```python
from build123d import *

# Parameters (mm, degrees)
STEEL_TUBE_STOCK_SKETCH_W        = 20
STEEL_TUBE_STOCK_SKETCH_H        = 55
STEEL_TUBE_STOCK_DEPTH           = 40
TUBE_INTERIOR_SKETCH_W           = 16
TUBE_INTERIOR_SKETCH_H           = 55.2
TUBE_INTERIOR_DEPTH              = 36
GUIDE_BUSH_CLEARANCE_1_SKETCH_R  = 6.2
GUIDE_BUSH_CLEARANCE_1_DEPTH     = 20.3
GUIDE_BUSH_CLEARANCE_2_SKETCH_R  = 6.2
GUIDE_BUSH_CLEARANCE_2_DEPTH     = 20.3
SCREW_THROUGH_CLEARANCE_SKETCH_R = 3.3
SCREW_THROUGH_CLEARANCE_DEPTH    = 20.3
SPRING_PIN_CLEARANCE_1_SKETCH_R  = 1.7
SPRING_PIN_CLEARANCE_1_DEPTH     = 2.2
SPRING_PIN_CLEARANCE_2_SKETCH_R  = 1.7
SPRING_PIN_CLEARANCE_2_DEPTH     = 2.2
SPRING_PIN_CLEARANCE_3_SKETCH_R  = 1.7
SPRING_PIN_CLEARANCE_3_DEPTH     = 2.2
CLAMP_BOLT_CLEARANCE_1_SKETCH_R  = 1.7
CLAMP_BOLT_CLEARANCE_1_DEPTH     = 2.3
CLAMP_BOLT_CLEARANCE_2_SKETCH_R  = 1.7
CLAMP_BOLT_CLEARANCE_2_DEPTH     = 2.3


with BuildPart() as part:
    # Steel tube stock sketch → Steel tube stock (new body)
    with BuildSketch(Plane.XY.offset(-29)):
        with Locations((39.708348754, -28.5)):
            Rectangle(STEEL_TUBE_STOCK_SKETCH_W, STEEL_TUBE_STOCK_SKETCH_H)
    extrude(amount=STEEL_TUBE_STOCK_DEPTH)

    # Tube interior sketch → Tube interior (cut)
    with BuildSketch(Plane.XY.offset(-27)):
        with Locations((39.708348754, -28.5)):
            Rectangle(TUBE_INTERIOR_SKETCH_W, TUBE_INTERIOR_SKETCH_H)
    extrude(amount=TUBE_INTERIOR_DEPTH, mode=Mode.SUBTRACT)

    # Guide bush clearance 1 sketch → Guide bush clearance 1 (cut)
    with BuildSketch(Plane(origin=(29.6, 0, 0), x_dir=(0, 0, -1), z_dir=(1, 0, 0))):
        with Locations((28, -9)):
            Circle(GUIDE_BUSH_CLEARANCE_1_SKETCH_R)
    extrude(amount=GUIDE_BUSH_CLEARANCE_1_DEPTH, mode=Mode.SUBTRACT)

    # Guide bush clearance 2 sketch → Guide bush clearance 2 (cut)
    with BuildSketch(Plane(origin=(29.6, 0, 0), x_dir=(0, 0, -1), z_dir=(1, 0, 0))):
        with Locations((28, -50)):
            Circle(GUIDE_BUSH_CLEARANCE_2_SKETCH_R)
    extrude(amount=GUIDE_BUSH_CLEARANCE_2_DEPTH, mode=Mode.SUBTRACT)

    # Screw through clearance sketch → Screw through clearance (cut)
    with BuildSketch(Plane(origin=(29.6, 0, 0), x_dir=(0, 0, -1), z_dir=(1, 0, 0))):
        with Locations(Location((19.5, -29, 0), (0, 0, 180))):
            Circle(SCREW_THROUGH_CLEARANCE_SKETCH_R)
    extrude(amount=SCREW_THROUGH_CLEARANCE_DEPTH, mode=Mode.SUBTRACT)

    # Spring pin clearance 1 sketch → Spring pin clearance 1 (cut)
    with BuildSketch(Plane.XY.offset(8.9)):
        with Locations((35.708348754, -12)):
            Circle(SPRING_PIN_CLEARANCE_1_SKETCH_R)
    extrude(amount=SPRING_PIN_CLEARANCE_1_DEPTH, mode=Mode.SUBTRACT)

    # Spring pin clearance 2 sketch → Spring pin clearance 2 (cut)
    with BuildSketch(Plane.XY.offset(8.9)):
        with Locations((35.708348754, -29)):
            Circle(SPRING_PIN_CLEARANCE_2_SKETCH_R)
    extrude(amount=SPRING_PIN_CLEARANCE_2_DEPTH, mode=Mode.SUBTRACT)

    # Spring pin clearance 3 sketch → Spring pin clearance 3 (cut)
    with BuildSketch(Plane.XY.offset(8.9)):
        with Locations((35.708348754, -46)):
            Circle(SPRING_PIN_CLEARANCE_3_SKETCH_R)
    extrude(amount=SPRING_PIN_CLEARANCE_3_DEPTH, mode=Mode.SUBTRACT)

    # Clamp bolt clearance 1 sketch → Clamp bolt clearance 1 (cut)
    with BuildSketch(Plane(origin=(47.6, 0, 0), x_dir=(0, 0, -1), z_dir=(1, 0, 0))):
        with Locations(Location((12, -19, 0), (0, 0, 180))):
            Circle(CLAMP_BOLT_CLEARANCE_1_SKETCH_R)
    extrude(amount=CLAMP_BOLT_CLEARANCE_1_DEPTH, mode=Mode.SUBTRACT)

    # Clamp bolt clearance 2 sketch → Clamp bolt clearance 2 (cut)
    with BuildSketch(Plane(origin=(47.6, 0, 0), x_dir=(0, 0, -1), z_dir=(1, 0, 0))):
        with Locations(Location((12, -39, 0), (0, 0, 180))):
            Circle(CLAMP_BOLT_CLEARANCE_2_SKETCH_R)
    extrude(amount=CLAMP_BOLT_CLEARANCE_2_DEPTH, mode=Mode.SUBTRACT)


with BuildPart() as body_2:
    # Mirror1: mirrored copy
    add(part.part.mirror(Plane(origin=(0, 0, 0), x_dir=(0, 0, 1), z_dir=(0, -1, 0))))


solid = body_2.part
```
Design review of the part built by this model. Coordinates are the model's own, in mm. A direction names the side the tool comes from. Round coordinates to 2 decimals unless told otherwise and drop trailing zeros. Write each loop counter-clockwise with the first axis right and the second up, starting at its lowest first coordinate (ties: lowest second). Pieces come first, ordered by that corner, then holes. Notation, with made-up numbers: (79.25, -23) -> (134.25, -23) arc R16 cw to (134.25, -10) -> close; hole circle Ø6 at (34, -13.75). An arc over 180 degrees is marked (long way). Answer in a Markdown table with one row per item.
Q1. Take a section at A-A, the plane z = -19.5. State the section outline as (x, y) points, then the cut area to 3 significant figures.
The answers:
| item | result |
|---|---|
| outline | (29.71, 1) -> (31.71, 1) -> (31.71, 25.7) -> (29.71, 25.7) -> close; (29.71, 32.3) -> (31.71, 32.3) -> (31.71, 56) -> (29.71, 56) -> close; (47.71, 1) -> (49.71, 1) -> (49.71, 25.7) -> (47.71, 25.7) -> close; (47.71, 32.3) -> (49.71, 32.3) -> (49.71, 56) -> (47.71, 56) -> close |
| area | 194 mm² |
Q2. Take a section at D-D, the plane y = 50. State the section outline as (x, z) points, then the cut area to 3 significant figures.
The answers:
| item | result |
|---|---|
| outline | (29.71, -21.8) -> (31.71, -21.8) -> (31.71, 9) -> (47.71, 9) -> (47.71, -21.8) -> (49.71, -21.8) -> (49.71, 11) -> (29.71, 11) -> close |
| area | 163 mm² |
Q3. Draft analysis for pull direction X (two halves, no side actions). For faces 4 (the face through (49.708, 29, -9)), 5 (the face through (30.7, 29.1, -22.8)), 6 (the face through (47.708, 29, -9)), state which applies: +X half, -X half, draft (parallel to the pull), parting line (faces both ways), or undercut.
The answers:
| item | result |
|---|---|
| face 4 | +X half |
| face 5 | draft |
| face 6 | undercut |
Q4. Clearance check with flat-ended pins moving along their axes: pin 1 Ø2 at (x, y) = (35.71, 12) entering from -Z; pin 2 Ø2.5 at (y, z) = (19, -12) entering from +X; pin 3 Ø1 at (x, y) = (45.5, 49) entering from -Z. State where each tip first meets the part, or that it passes through.
The answers:
| item | result |
|---|---|
| pin 1 | through |
| pin 2 | x = 31.71 |
| pin 3 | z = 9 |
Q5. Take a section at B-B, the plane z = -1. State the section outline as (x, y) points, then the cut area to 3 significant figures.
The answers:
| item | result |
|---|---|
| outline | (29.71, 1) -> (31.71, 1) -> (31.71, 56) -> (29.71, 56) -> close; (47.71, 1) -> (49.71, 1) -> (49.71, 56) -> (47.71, 56) -> close |
| area | 220 mm² |
Q6. Take a section at C-C, the plane x = 45.5. State the section outline as (y, z) points, then the cut area to 3 significant figures.
The answers:
| item | result |
|---|---|
| outline | (1, -29) -> (2.88, -29) arc R6.2 cw to (2.88, -27) -> (1, -27) -> close; (1, 9) -> (56, 9) -> (56, 11) -> (1, 11) -> close; (15.12, -29) -> (43.88, -29) arc R6.2 cw to (43.88, -27) -> (15.12, -27) arc R6.2 cw to start |
| area | 171 mm² |
Q7. To check wall thickness, follow L1, parallel to X at y = 15.5, z = -16; L2, parallel to Z at x = 39.5, y = 24; L3, parallel to Y at x = 48.6, z = -12. State the ranges of each line that lie inside material, in increasing order. Write a range as [from, to].
The answers:
| item | result |
|---|---|
| L1 | [29.71, 31.71], [47.71, 49.71] |
| L2 | [-29, -27], [9, 11] |
| L3 | [1, 17.3], [20.7, 37.3], [40.7, 56] |
Q8. For faces 1 (the face through (48.7, 29.1, -22.8)), 2 (the face through (48.69, 19.51, -10.38)), 3 (the face through (40, 28, 9)), list the 3-axis set-ups (+Z, -Z, +X, -X, +Y, -Y) from which the entire face can be reached by the end or side of a thin tool; tool diameter is ignored.
The answers:
| item | result |
|---|---|
| face 1 | +X, -X |
| face 2 | +X |
| face 3 | +Y, -Y |
